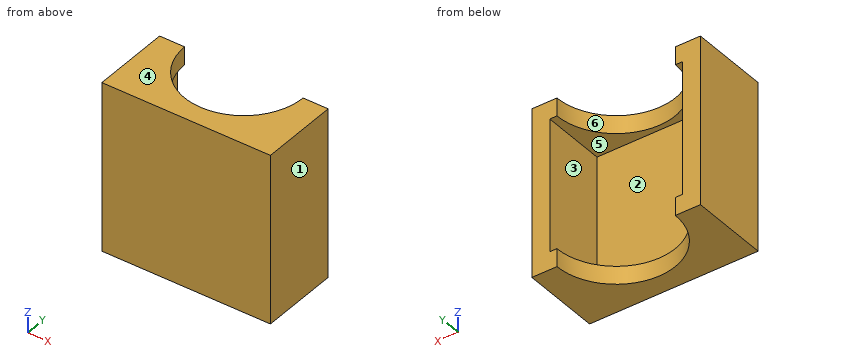
```python
from build123d import *

# Parameters (mm, degrees)
SKETCH1_W           = 74.6125
SKETCH1_H           = 74.6125
BOSS_EXTRUDE1_DEPTH = 34.925
SKETCH2_R           = 26.19375
CUT_EXTRUDE1_DEPTH  = 91.435264528
SKETCH3_W           = 58.7375
SKETCH3_H           = 58.7375
CUT_EXTRUDE2_DEPTH  = 28.575


with BuildPart() as part:
    # Sketch1 → Boss-Extrude1 (new body)
    with BuildSketch(Plane(origin=(0, 0, 0), x_dir=(1, 0, 0), z_dir=(0, 1, 0))):
        Rectangle(SKETCH1_W, SKETCH1_H)
    extrude(amount=BOSS_EXTRUDE1_DEPTH)

    # Sketch2 → Cut-Extrude1 (cut, through all)
    with BuildSketch(Plane.XY.offset(37.30625)):
        with Locations((0, 34.925)):
            Circle(SKETCH2_R)
    extrude(amount=-CUT_EXTRUDE1_DEPTH, mode=Mode.SUBTRACT)

    # Sketch3 → Cut-Extrude2 (cut)
    with BuildSketch(Plane(origin=(0, 34.925, 0), x_dir=(1, 0, 0), z_dir=(0, 1, 0))):
        Rectangle(SKETCH3_W, SKETCH3_H)
    extrude(amount=-CUT_EXTRUDE2_DEPTH, mode=Mode.SUBTRACT)


solid = part.part
```
Geometry check sheet. Reference: the model listing, model coordinates, mm. Face numbers are marked on the shaded views. A direction names the side the tool comes from. Give positions to 0.01 mm unless a question says otherwise; leave off trailing zeros. Write each loop counter-clockwise with the first axis right and the second up, starting at its lowest first coordinate (ties: lowest second). Pieces come first, ordered by that corner, then holes. Notation, with made-up numbers: (2, 47.25) - (38, 47.25) arc R24 cw to (38, 69.25) - close; hole circle Ø5 at (-31, -16). An arc over 180 degrees is marked (long way). Use a Markdown table: item, result.
Q1. Set-up check for the marked faces 1 and 2: record each of +Z, -Z, +X, -X, +Y, -Y from which the full face is reachable in a straight line by a thin tool's end or side.
Computed:
| item | result |
|---|---|
| face 1 | +Z, -Z, +X, +Y, -Y |
| face 2 | +Y |
Q2. Section check A-A, the plane z = 26. Enter the section's corners in (x, y) (3 decimals).
Computed:
| item | result |
|---|---|
| outline | (-37.306, 0) - (37.306, 0) - (37.306, 34.925) - (29.369, 34.925) - (29.369, 6.35) - (-29.369, 6.35) - (-29.369, 34.925) - (-37.306, 34.925) - close |
Q3. Section check B-B, the plane y = 33.5. Enter the section's corners in (x, z).
Computed:
| item | result |
|---|---|
| outline | (-37.31, -37.31) - (-26.15, -37.31) - (-26.15, -29.37) - (-29.37, -29.37) - (-29.37, 29.37) - (-26.15, 29.37) - (-26.15, 37.31) - (-37.31, 37.31) - close; (26.15, -37.31) - (37.31, -37.31) - (37.31, 37.31) - (26.15, 37.31) - (26.15, 29.37) - (29.37, 29.37) - (29.37, -29.37) - (26.15, -29.37) - close |
Q4. Section check C-C, the plane x = 13.5. Enter the section's corners in (y, z).
Computed:
| item | result |
|---|---|
| outline | (0, -37.31) - (12.48, -37.31) - (12.48, -29.37) - (6.35, -29.37) - (6.35, 29.37) - (12.48, 29.37) - (12.48, 37.31) - (0, 37.31) - close |
Q5. Thickness scan on L1, parallel to Z at x = 28, y = 10.5; L2, parallel to Y at x = 8, z = -6.5. Record the ranges inside material, lowest first. Write a range as [from, to].
Computed:
| item | result |
|---|---|
| L1 | z = [-37.31, -29.37], [29.37, 37.31] |
| L2 | y = [0, 6.35] |
Q6. Draft check along Z on the marked faces 3, 4, 5 and 6. Enter one of: pulls with the +Z half, pulls with the -Z half, needs draft (parallel to the pull), parting line crosses it, or undercut.
Computed:
| item | result |
|---|---|
| face 3 | undercut |
| face 4 | pulls with the +Z half |
| face 5 | undercut |
| face 6 | needs draft |
Q7. Section check D-D, the plane y = 28.5. Enter the section's corners in (x, z), then the cut area to 3 significant figures.
Computed:
| item | result |
|---|---|
| outline | (-37.31, -37.31) - (-25.39, -37.31) - (-25.39, -29.37) - (-29.37, -29.37) - (-29.37, 29.37) - (-25.39, 29.37) - (-25.39, 37.31) - (-37.31, 37.31) - close; (25.39, -37.31) - (37.31, -37.31) - (37.31, 37.31) - (25.39, 37.31) - (25.39, 29.37) - (29.37, 29.37) - (29.37, -29.37) - (25.39, -29.37) - close |
| area | 1,310 mm² |
Q8. Go/stop test with flat-tipped pins: P1, Ø14.5, axis at x = -9, y = 22.5, coming from the -Z side; P2, Ø17.5, axis at x = -6.5, z = -8, coming from the +Y side. Record where each tip stops, or that it passes through.
Computed:
| item | result |
|---|---|
| P1 | passes through |
| P2 | stops at y = 6.35 |
